Build history of the part. All positions in model axes, mm. A direction names the side the tool comes from. Round coordinates to 2 decimals unless told otherwise and drop trailing zeros. Write each loop counter-clockwise with the first axis right and the second up, starting at its lowest first coordinate (ties: lowest second). Pieces come first, ordered by that corner, then holes.
from build123d import *

# Parameters (mm, degrees)
F2_R     = 1.9304
F3_DEPTH = 12.7
F4_R     = 1.4224
F5_DEPTH = 12.7


with BuildPart() as f1:
    # F0 (on Right) → F1 (revolve)
    with BuildSketch(Plane.YZ):
        Polygon((0, 2.032), (0, 0), (83.178809, 0), (83.178809, 1.524), (57.778809, 1.524), (51.101475, 5), (31.101475, 5), (25.4, 2.032), align=None)
    revolve(axis=Axis((0, 41.589404, 0), (0, 1, 0)))

    # F2 (on face) → F3 (cut)
    with BuildSketch(Plane.XZ):
        Circle(F2_R)
    extrude(amount=-F3_DEPTH, mode=Mode.SUBTRACT)

    # F4 (on face) → F5 (cut)
    with BuildSketch(Plane(origin=(0, 83.178809, 0), x_dir=(-1, 0, 0), z_dir=(0, 1, 0))):
        Circle(F4_R)
    extrude(amount=-F5_DEPTH, mode=Mode.SUBTRACT)


solid = f1.part
1) Wall check: L1, parallel to X at y = 61, z = -0.5; L2, parallel to Y at x = -0.5, z = -0.25; L3, parallel to Z at x = -1.25, y = 77.5. Give the ranges that are in metal, low to high.
Results:
L1: x = -1.44 to 1.44
L2: y = 12.7 to 70.48
L3: z = -0.87 to -0.68, 0.68 to 0.87
2) Slice it at C-C (y = 19). Write the cut outline in (x, z).
Results:
outline: circle Ø4.06 at (0, 0)
3) Slice it at D-D (y = 78). Write the cut outline in (x, z).
Results:
outline: circle Ø3.05 at (0, 0); hole circle Ø2.84 at (0, 0)
4) Slice it at A-A (x = 0). Write the cut outline in (y, z).
Results:
outline: (0, -2.03) - (25.4, -2.03) - (31.1, -5) - (51.1, -5) - (57.78, -1.52) - (83.18, -1.52) - (83.18, -1.42) - (70.48, -1.42) - (70.48, 1.42) - (83.18, 1.42) - (83.18, 1.52) - (57.78, 1.52) - (51.1, 5) - (31.1, 5) - (25.4, 2.03) - (0, 2.03) - (0, 1.93) - (12.7, 1.93) - (12.7, -1.93) - (0, -1.93) - close
5) Which spindle directions (+Z, -Z, +X, -X, +Y, -Y) get a long thin tool onto all of the face, cutting with end or side? Do faces 1 (the flat face through (0, 70.479, 0)), 2 (the cylindrical face through (-4.88, 40.96, -1.08)). Say none if no direction does.
Results:
face 1: +Y
face 2: +Y, -Y
6) Mould opens along Z. For faces 3 (the flat face through (0, 12.7, 0)), 4 (the conical face through (-2.768, 26.944, -0.615)) say: released by +Z, released by -Z, zero draft, split by the parting line, or undercut.
Results:
face 3: undercut
face 4: split by the parting line
7) Pin check, flat tips, straight feed: pin 1 Ø2 at (x, y) = (2, 72.5) entering from -Z; pin 2 Ø1.5 at (x, z) = (2, -2.5) entering from -Y; pin 3 Ø1.5 at (x, z) = (-2, 2.5) entering from +Y. Stop position of each tip, or through.
Results:
pin 1: stops at z = -1.15
pin 2: stops at y = 26.21
pin 3: stops at y = 56
8) Slice it at B-B (z = 0). Write the cut outline in (x, y).
Results:
outline: (-5, 31.1) - (-2.03, 25.4) - (-2.03, 0) - (-1.93, 0) - (-1.93, 12.7) - (1.93, 12.7) - (1.93, 0) - (2.03, 0) - (2.03, 25.4) - (5, 31.1) - (5, 51.1) - (1.52, 57.78) - (1.52, 83.18) - (1.42, 83.18) - (1.42, 70.48) - (-1.42, 70.48) - (-1.42, 83.18) - (-1.52, 83.18) - (-1.52, 57.78) - (-5, 51.1) - close
